Work out the finished part from the listing and answer in its coordinate system (mm). A direction names the side the tool comes from. Coordinates: 2 decimals unless noted, no trailing zeros. Write each loop counter-clockwise with the first axis right and the second up, starting at its lowest first coordinate (ties: lowest second). Pieces come first, ordered by that corner, then holes. Notation, with made-up numbers: (40, 48) - (80, 48) arc R13 ccw to (80, 52) - close; hole circle Ø6 at (-33.5, 14.5). An arc over 180 degrees is marked (long way). Use one line per item in the form item = value. Start each with the question number.
Item 1: Given pin 1 (1.5 mm diameter, centred on x = -19.5, z = -15, fed in from +Y); pin 2 (1.2 mm diameter, centred on x = -19.1, z = 14.575, fed in from -Y), each flat-ended and moving along its own axis, determine where each tip first touches the part or whether it passes through.
Item 2: Consider probe 1 along Z at (x, y) = (-19.1, 1.6) (3 decimals); probe 2 along Z at (x, y) = (19.1, 0.9) (3 decimals); probe 3 along Z at (x, y) = (6, 6). Determine where each line is inside the solid, lowest interval first.
Item 3: A cutting plane is placed at D-D (y = 0.5). Write down the section's boundary in (x, z) (3 decimals).
Item 4: A cutting plane is placed at C-C (x = 19.1). Write down the section's boundary in (y, z) (3 decimals).
Item 5: Determine the mould class of faces 1 (the flat face through (-22.1, 4, 0)), 2 (the flat face through (0, 4, 19.4)), 3 (the flat face through (0, 4, -19.4)) for opening direction Z: released by +Z, released by -Z, zero draft, split by the parting line, or undercut.
Item 6: For faces 4 (the flat face through (23.1, 4, 0)), 5 (the flat face through (19, 4, 16)), 6 (the flat face through (-16.506, 0.5, 0.2)), determine the directions among +Z, -Z, +X, -X, +Y, -Y from which every point of the face is accessible in a straight line to the end or side of a thin tool.
Item 7: A cutting plane is placed at B-B (x = -6). Write down the section's boundary in (y, z).
Item 8: A cutting plane is placed at A-A (z = -7). Write down the section's boundary in (x, y).
Autodesk Fusion 360 part; units mm, degrees
sketch "Sketch1" plane through (0, 0, 0) normal (0, 1, 0) x (1, 0, 0)
  line L0 (19.1, 14.575) -> (-19.1, 14.575) construction
  line L1 (-19.1, 14.575) -> (-19.1, -14.575) construction
  line L2 (-19.1, -14.575) -> (19.1, -14.575) construction
  line L3 (19.1, -14.575) -> (19.1, 14.575) construction
  line L4 (19.1, 14.575) -> (-19.1, -14.575) construction
  line L5 (-19.1, 14.575) -> (19.1, -14.575) construction
  circle A0 centre (-19.1, 14.575) radius 1
  circle A1 centre (19.1, 14.575) radius 1
  circle A2 centre (-19.1, -14.575) radius 1
  circle A3 centre (19.1, -14.575) radius 1
  circle A4 centre (-19.1, 14.575) radius 2.5
  circle A5 centre (19.1, 14.575) radius 2.5
  circle A6 centre (-19.1, -14.575) radius 2.5
  circle A7 centre (19.1, -14.575) radius 2.5
  line L6 (22.1, -18.4) -> (-22.1, -18.4)
  line L7 (-22.1, -18.4) -> (-22.1, 18.4)
  line L8 (-22.1, 18.4) -> (22.1, 18.4)
  line L9 (22.1, 18.4) -> (22.1, -18.4)
  line L10 (22.1, -18.4) -> (-22.1, 18.4) construction
  line L11 (-22.1, -18.4) -> (22.1, 18.4) construction
  line L12 (23.1, 19.4) -> (-23.1, 19.4)
  line L13 (-23.1, 19.4) -> (-23.1, -19.4)
  line L14 (-23.1, -19.4) -> (23.1, -19.4)
  line L15 (23.1, -19.4) -> (23.1, 19.4)
  line L16 (23.1, 19.4) -> (-23.1, -19.4) construction
  line L17 (-23.1, 19.4) -> (23.1, -19.4) construction
  line L18 (-16.5064, 18.4) -> (16.5064, 18.4)
  line L19 (16.5064, 18.4) -> (16.5064, -18.4)
  line L20 (16.5064, -18.4) -> (-16.5064, -18.4)
  line L21 (-16.5064, -18.4) -> (-16.5064, 18.4)
  line L22 (-16.5064, 18.4) -> (16.5064, -18.4) construction
  line L23 (16.5064, 18.4) -> (-16.5064, -18.4) construction
  line L24 (22.1, 11.9339) -> (-22.1, 11.9339)
  line L25 (-22.1, 11.9339) -> (-22.1, -11.9339)
  line L26 (-22.1, -11.9339) -> (22.1, -11.9339)
  line L27 (22.1, -11.9339) -> (22.1, 11.9339)
  line L28 (22.1, 11.9339) -> (-22.1, -11.9339) construction
  line L29 (-22.1, 11.9339) -> (22.1, -11.9339) construction
  dimension "d1" = 29.15
  dimension "d2" = 38.2
  dimension "d3" = 2
  dimension "d4" = 2
  dimension "d5" = 2
  dimension "d6" = 2
  dimension "d7" = 5
  dimension "d8" = 5
  dimension "d9" = 5
  dimension "d10" = 5
  dimension "d11" = 36.8
  dimension "d12" = 1
  dimension "d13" = 1
  dimension "d14" = 44.2
extrude "Extrude1" add sketch "Sketch1" along normal blind 8 contours L12 L13 L14 L15 makes body 1
extrude "Extrude2" add sketch "Sketch1" along normal blind 4 separate body contours A4 | A5 | A6 | A7 makes body 2 at (21.5969, 2.6667, -14.4504) makes body 3 at (-16.6031, 2.6667, 14.6996) makes body 4 at (-16.6031, 2.6667, -14.4504) makes body 5 at (21.5969, 2.6667, 14.6996)
extrude "Extrude3" add sketch "Sketch1" along normal blind 1 contours L6 L9 L19 L26 | L6 L19 L20 L21 L26 | L9 L19 L24 L26 L27 | L6 L7 L21 L26 | L8 L9 L19 L24 | L7 L21 L24 L25 L26 | L8 L18 L19 L21 L24 | L7 L8 L21 L24 bodies 1 2 3 4 5
Answer:
q1.pin_1 = 4
q1.pin_2 = through
q2.probe_1 = -19.4 to -18.4, -17.075 to -15.575, -13.575 to -12.075, 12.075 to 13.575, 15.575 to 17.075, 18.4 to 19.4
q2.probe_2 = -19.4 to -15.575, -13.575 to 13.575, 15.575 to 19.4
q2.probe_3 = -19.4 to -18.4, 18.4 to 19.4
q3.outline = (-23.1, -19.4) - (23.1, -19.4) - (23.1, 19.4) - (-23.1, 19.4) - close; hole circle Ø2 at (-19.1, -14.575); hole circle Ø2 at (-19.1, 14.575); hole (-16.506, -11.934) - (16.506, -11.934) - (16.506, 11.934) - (-16.506, 11.934) - close; hole circle Ø2 at (19.1, -14.575); hole circle Ø2 at (19.1, 14.575)
q4.outline = (0, -19.4) - (8, -19.4) - (8, -18.4) - (1, -18.4) - (1, -17.075) - (4, -17.075) - (4, -15.575) - (0, -15.575) - close; (0, -13.575) - (4, -13.575) - (4, -12.075) - (1, -12.075) - (1, 12.075) - (4, 12.075) - (4, 13.575) - (0, 13.575) - close; (0, 15.575) - (4, 15.575) - (4, 17.075) - (1, 17.075) - (1, 18.4) - (8, 18.4) - (8, 19.4) - (0, 19.4) - close
q5.face_1 = undercut
q5.face_2 = released by +Z
q5.face_3 = released by -Z
q6.face_4 = +Z, -Z, +X, +Y, -Y
q6.face_5 = +Y
q6.face_6 = +Y, -Y
q7.outline = (0, -19.4) - (8, -19.4) - (8, -18.4) - (1, -18.4) - (1, -11.93) - (0, -11.93) - close; (0, 11.93) - (1, 11.93) - (1, 18.4) - (8, 18.4) - (8, 19.4) - (0, 19.4) - close
q8.outline = (-23.1, 0) - (-16.51, 0) - (-16.51, 1) - (-22.1, 1) - (-22.1, 8) - (-23.1, 8) - close; (16.51, 0) - (23.1, 0) - (23.1, 8) - (22.1, 8) - (22.1, 1) - (16.51, 1) - close
